from build123d import *

# Parameters (mm, degrees)
WALL_DEPTH                = 19.05
ROOF_START                = 19.05
ROOF_DEPTH                = 3.175
F_2_56_TAPPED_HOLE1_D     = 1.778
F_2_56_TAPPED_HOLE1_DEPTH = 5.73
F_2_56_TAPPED_HOLE1_TIP   = 0.53416509
BOSS_EXTRUDE1_DEPTH       = 1.5875
FILLET1_R                 = 1.5875


with BuildPart() as part:
    # MainSketch → Wall (new body)
    with BuildSketch(Plane(origin=(0, 0, 0), x_dir=(1, 0, 0), z_dir=(0, 1, 0))):
        Polygon((-32.75, -4), (0, -4), (0, 0), (-36.75, 0), (-36.75, -45.5), (0, -45.5), (0, -41.5), (-32.75, -41.5), align=None)
    extrude(amount=WALL_DEPTH)

    # MainSketch<3> → Roof (add)
    with BuildSketch(Plane(origin=(0, 0, 0), x_dir=(1, 0, 0), z_dir=(0, 1, 0)).offset(ROOF_START)):
        with BuildLine():
            Line((0, -21.625), (0, 0))
            Line((0, 0), (-36.75, 0))
            Line((-36.75, 0), (-36.75, -45.5))
            Line((-36.75, -45.5), (0, -45.5))
            Line((0, -45.5), (0, -23.875))
            ThreePointArc((0, -23.875), (-0.353553391, -23.728553391), (-0.5, -23.375))
            Line((-0.5, -23.375), (-0.5, -22.125))
            ThreePointArc((-0.5, -22.125), (-0.353553391, -21.771446609), (0, -21.625))
        make_face()
    extrude(amount=ROOF_DEPTH)

    # #2-56 Tapped Hole1
    with Locations(Plane(origin=(-18.375, 0, 43), x_dir=(0, 0, -1), z_dir=(0, -1, 0))):
        with Locations((0, 0), (40.5, 0)):
            Hole(F_2_56_TAPPED_HOLE1_D / 2, depth=F_2_56_TAPPED_HOLE1_DEPTH)
            with Locations((0, 0, -(F_2_56_TAPPED_HOLE1_DEPTH + F_2_56_TAPPED_HOLE1_TIP / 2))):  # 118° drill point
                Cone(0, F_2_56_TAPPED_HOLE1_D / 2, F_2_56_TAPPED_HOLE1_TIP, mode=Mode.SUBTRACT)

    # Sketch3 → Boss-Extrude1 (add)
    with BuildSketch(Plane(origin=(0, 0, 0), x_dir=(0, 0, -1), z_dir=(1, 0, 0))):
        Polygon((-44, 21.1375), (-44, 0), (-43, 0), (-43, 20.1375), (-24.875, 20.1375), (-24.875, 21.1375), align=None)
        Polygon((-1.5, 21.1375), (-20.625, 21.1375), (-20.625, 20.1375), (-2.5, 20.1375), (-2.5, 0), (-1.5, 0), align=None)
    extrude(amount=BOSS_EXTRUDE1_DEPTH)

    # Fillet1
    fillet1_edges = [part.edges().sort_by_distance(p)[0] for p in [
        (0.79375, 20.1375, 43),
        (0.79375, 21.1375, 44),
        (0.79375, 20.1375, 2.5),
        (0.79375, 21.1375, 1.5),
        (1.5875, 20.6375, 20.625),
        (1.5875, 20.6375, 24.875),
    ]]
    fillet(fillet1_edges, radius=FILLET1_R - 0.0001)  # a hair under: the kernel refuses the full size


solid = part.part
Verification items for the finished model (mm, model axes). A direction names the side the tool comes from. Coordinates: 2 decimals unless noted, no trailing zeros. Order: outer loops, then holes, each group sorted by start corner. A loop starts at its lowest first (then second) coordinate and runs counter-clockwise, first axis right, second up. Notation, with made-up numbers: M -4.75,63 L 25.25,63 A24 cw 25.25,90 Z; hole C 48.5,19 d10. An arc over 180 degrees is marked long. One line per item, written item: value. Start each with the question number.
Item 1: Sectioned sample at A-A on y = 10.5. Record the cut outline in (x, z), then the cut area to 3 significant figures.
Item 2: Access from +Z, -Z, +X, -X, +Y, -Y to the whole of each face (thin tool, end or side, straight path). Record for faces 5 (the flat face through (0, 14, 42)), 6 (the flat face through (1, 20.138, 12)), 7 (the flat face through (-0.5, 21, 23)), 8 (the cylindrical face through (-17.494, 2.905, 2.384)).
Item 3: Depth check by flat-ended pin: P1, Ø1.3, axis at x = 1, z = 10.5, coming from the -Y side; P2, Ø4, axis at x = -30.5, z = 37.5, coming from the -Y side; P3, Ø0.8, axis at x = 1, y = 5.5, coming from the +Z side. Enter the tip coordinate at first touch or a pass-through.
Item 4: Mould release check, pull along Z, two halves, no side actions. Record for faces 1 (the flat face through (1, 21.138, 34)), 2 (the cylindrical face through (1.11, 20.63, 20.17)), 3 (the cylindrical face through (0.805, 20.685, 1.977)), 4 (the cylindrical face through (0.8, 20.66, 43.55)): pulls with the +Z half, pulls with the -Z half, needs draft (parallel to the pull), parting line crosses it, or undercut.
Item 5: Sectioned sample at C-C on x = -23. Record the cut outline in (y, z) (3 decimals).
Item 6: Thickness scan on probe 1 along Z at (x, y) = (-23.5, 10.25); probe 2 along Z at (x, y) = (-18, 5.75); probe 3 along X at (y, z) = (1.25, 37). Record the ranges inside material, lowest first.
Calculated:
1. outline: M -36.75,0 L 0,0 L 0,1.5 L 1.59,1.5 L 1.59,2.5 L 0,2.5 L 0,4 L -32.75,4 L -32.75,41.5 L 0,41.5 L 0,43 L 1.59,43 L 1.59,44 L 0,44 L 0,45.5 L -36.75,45.5 Z
1. area: 447 mm^2
2. face 5: +X
2. face 6: +X, -Y
2. face 7: +X, +Y, -Y
2. face 8: -Y
3. P1: y = 20.14
3. P2: y = 19.05
3. P3: z = 44
4. face 1: needs draft
4. face 2: undercut
4. face 3: pulls with the -Z half
4. face 4: pulls with the +Z half
5. outline: M 0,0 L 22.225,0 L 22.225,45.5 L 0,45.5 L 0,41.5 L 19.05,41.5 L 19.05,4 L 0,4 Z
6. probe 1: 0 to 4, 41.5 to 45.5
6. probe 2: 0 to 1.73, 3.27 to 4, 41.5 to 42.23, 43.77 to 45.5
6. probe 3: -36.75 to -32.75
